The listing builds one solid part. Answer for the finished solid, in the listing's coordinates (mm). Give positions to 0.01 mm unless a question says otherwise; leave off trailing zeros. Loops run counter-clockwise (first coordinate to the right, second up) from the corner with the lowest first, then second, coordinate; pieces in that order, holes last. Notation, with made-up numbers: (0, -0.5) - (34, -0.5) arc R22 cw to (34, 16.5) - close; hole circle Ø8 at (14, 42.5). An arc over 180 degrees is marked (long way). One line per item, written item: value. Start each with the question number.
from build123d import *

# Parameters (mm, degrees)
BOSS_EXTRUDE1_DEPTH = 3.0099
BOSS_EXTRUDE2_DEPTH = 6.0198
CRVPATTERN1_START   = -3.0099
CRVPATTERN1_DEPTH   = 6.0198


# Read off the part's stored shape, not the designer's step: CrvPattern1
with BuildPart() as part:
    # Sketch1 → Boss-Extrude1 (new, symmetric)
    with BuildSketch(Plane(origin=(0, 0, 0), x_dir=(1, 0, 0), z_dir=(0, 1, 0))):
        with BuildLine():
            Line((0, -6), (0, -6.635))
            ThreePointArc((0, -6.635), (-6.635, 0), (0, 6.635))
            Line((0, 6.635), (0, 6))
            ThreePointArc((0, 6), (-6, 0), (0, -6))
        make_face()
    extrude(amount=BOSS_EXTRUDE1_DEPTH, both=True)

    # Sketch2 → Boss-Extrude2 (add)
    with BuildSketch(Plane(origin=(0, 3.0099, 0), x_dir=(1, 0, 0), z_dir=(0, 1, 0))):
        with BuildLine():
            Line((0, -6), (-0.097943085, -5.475567721))
            ThreePointArc((-0.097943085, -5.475567721), (-0.413392769, -5.191665428), (-0.769794827, -5.422070697))
            Line((-0.769794827, -5.422070697), (-0.949494698, -5.924395312))
            ThreePointArc((-0.949494698, -5.924395312), (-0.47625, -5.981068963), (0, -6))
        make_face()
    extrude(amount=-BOSS_EXTRUDE2_DEPTH)

    # CrvPattern1 outline → CrvPattern1 (add)
    with BuildSketch(Plane(origin=(0, 0, 0), x_dir=(1, 0, 0), z_dir=(0, 1, 0)).offset(CRVPATTERN1_START)):
        with BuildLine():
            ThreePointArc((-1.392781631, -5.296375557), (-1.631964533, -4.945803803), (-2.0328165, -5.085183555))
            Line((-2.0328165, -5.085183555), (-2.326440816, -5.530612365))
            ThreePointArc((-2.326440816, -5.530612365), (-1.880108137, -5.697823566), (-1.421911325, -5.829079531))
            Line((-1.421911325, -5.829079531), (-1.392781631, -5.296375557))
        make_face()
        with BuildLine():
            ThreePointArc((-0.667838723, 5.962716784), (-1.139022221, 5.890893683), (-1.603018095, 5.781897006))
            Line((-1.603018095, 5.781897006), (-1.368522884, 5.302695525))
            ThreePointArc((-1.368522884, 5.302695525), (-0.988689868, 5.113391814), (-0.706800505, 5.430641561))
            Line((-0.706800505, 5.430641561), (-0.667838723, 5.962716784))
        make_face()
        with BuildLine():
            ThreePointArc((-2.061889926, 5.634590485), (-2.502629927, 5.453149865), (-2.927577467, 5.237297984))
            Line((-2.927577467, 5.237297984), (-2.586198593, 4.827319293))
            ThreePointArc((-2.586198593, 4.827319293), (-2.172323601, 4.733423039), (-1.97364785, 5.108438987))
            Line((-1.97364785, 5.108438987), (-2.061889926, 5.634590485))
        make_face()
        with BuildLine():
            ThreePointArc((-3.338468064, 4.985441905), (-3.723654071, 4.704721071), (-4.085342534, 4.394311821))
            Line((-4.085342534, 4.394311821), (-3.656529542, 4.076913836))
            ThreePointArc((-3.656529542, 4.076913836), (-3.232192478, 4.083774637), (-3.128049589, 4.495190818))
            Line((-3.128049589, 4.495190818), (-3.338468064, 4.985441905))
        make_face()
        with BuildLine():
            ThreePointArc((-4.424842028, 4.052255302), (-4.732528651, 3.6882479), (-5.010351382, 3.300966378))
            Line((-5.010351382, 3.300966378), (-4.518535244, 3.09423237))
            ThreePointArc((-4.518535244, 3.09423237), (-4.10791207, 3.201459343), (-4.104235427, 3.625835941))
            Line((-4.104235427, 3.625835941), (-4.424842028, 4.052255302))
        make_face()
        with BuildLine():
            ThreePointArc((-5.2591173, 2.888197574), (-5.471774558, 2.461642376), (-5.649903027, 2.019553363))
            Line((-5.649903027, 2.019553363), (-5.123104226, 1.93526169))
            ThreePointArc((-5.123104226, 1.93526169), (-4.749589577, 2.136745739), (-4.846588652, 2.549904539))
            Line((-4.846588652, 2.549904539), (-5.2591173, 2.888197574))
        make_face()
        with BuildLine():
            ThreePointArc((-5.793762308, 1.559589152), (-5.899274375, 1.094788495), (-5.967559981, 0.623079345))
            Line((-5.967559981, 0.623079345), (-5.435792082, 0.666032397))
            ThreePointArc((-5.435792082, 0.666032397), (-5.120666391, 0.950294273), (-5.312814808, 1.328696177))
            Line((-5.312814808, 1.328696177), (-5.793762308, 1.559589152))
        make_face()
        with BuildLine():
            ThreePointArc((-5.998316459, 0.142125493), (-5.990671945, -0.334439306), (-5.945224219, -0.808893678))
            Line((-5.945224219, -0.808893678), (-5.438783895, -0.641143085))
            ThreePointArc((-5.438783895, -0.641143085), (-5.200000973, -0.290298773), (-5.476351366, 0.031787357))
            Line((-5.476351366, 0.031787357), (-5.998316459, 0.142125493))
        make_face()
        with BuildLine():
            ThreePointArc((-5.861125591, -1.28343555), (-5.740760029, -1.744612933), (-5.584168287, -2.194781205))
            Line((-5.584168287, -2.194781205), (-5.131909211, -1.911790408))
            ThreePointArc((-5.131909211, -1.911790408), (-4.983073354, -1.514352485), (-5.327881076, -1.266932499))
            Line((-5.327881076, -1.266932499), (-5.861125591, -1.28343555))
        make_face()
        with BuildLine():
            ThreePointArc((-5.390005944, -2.635874792), (-5.163776982, -3.055389873), (-4.904962802, -3.455624388))
            Line((-4.904962802, -3.455624388), (-4.532651751, -3.073516361))
            ThreePointArc((-4.532651751, -3.073516361), (-4.482242656, -2.652128252), (-4.875862809, -2.49347079))
            Line((-4.875862809, -2.49347079), (-5.390005944, -2.635874792))
        make_face()
        with BuildLine():
            ThreePointArc((-4.611798851, -3.838139049), (-4.292595541, -4.19209059), (-3.94630447, -4.519588591))
            Line((-3.94630447, -4.519588591), (-3.675153304, -4.060133361))
            ThreePointArc((-3.675153304, -4.060133361), (-3.726042954, -3.638803018), (-4.146049624, -3.577947349))
            Line((-4.146049624, -3.577947349), (-4.611798851, -3.838139049))
        make_face()
        with BuildLine():
            ThreePointArc((-3.570841484, -4.821731131), (-3.176849953, -5.089953278), (-2.762811401, -5.326056061))
            Line((-2.762811401, -5.326056061), (-2.608268548, -4.815430396))
            ThreePointArc((-2.608268548, -4.815430396), (-2.757557583, -4.418162477), (-3.180021524, -4.458575762))
            Line((-3.180021524, -4.458575762), (-3.570841484, -4.821731131))
        make_face()
    extrude(amount=CRVPATTERN1_DEPTH)


solid = part.part
1. Find the intervals of material crossed by L1, parallel to X at y = -1, z = 5.25; L2, parallel to Z at x = -4.5, y = -2; L3, parallel to Z at x = -3.75, y = 1.75, in increasing order. Write a range as [from, to].
2. A cutting plane is placed at A-A (z = -2.75). Determine the outline of the cut face in (x, y).
3. A flat-ended cylindrical pin translates along its axis: pin 1 (1 mm diameter, centred on x = -1, y = -2.5, fed in from +Z). Find the tip coordinate at first contact, or state that the pin passes through.
Results below:
1. L1: x = [-4.06, -2.74], [-2.14, -1.39], [-0.64, -0.25]
1. L2: z = [-4.88, -3.09], [2.63, 3.03], [3.78, 4.88]
1. L3: z = [-5.47, -4.15], [3.62, 4.19], [4.68, 5.47]
2. outline: (-6.04, -3.01) - (-5.09, -3.01) - (-5.09, 3.01) - (-6.04, 3.01) - close
3. pin 1: stops at z = 6.62
